The listing builds one solid part. Answer for the finished solid, in the listing's coordinates (mm). A direction names the side the tool comes from. Coordinates: 2 decimals unless noted, no trailing zeros. Order: outer loops, then holes, each group sorted by start corner. A loop starts at its lowest first (then second) coordinate and runs counter-clockwise, first axis right, second up. Notation, with made-up numbers: M 16.25,-16.75 L 36.25,-16.75 A16 cw 36.25,-11.75 Z; hole C 60,-1.5 d4. An arc over 180 degrees is marked long. One line per item, written item: value. Start each with the question number.
Q1. The part is cut by section B-B on y = 0. Give the number of separate pieces and of enclosed holes in the cut face, then the cut area to 3 significant figures.
Q2. Straight lines are drawn through the part: line 1 along X through (y, z) = (-0.25, 4.25); line 2 along X through (y, z) = (0, 1.15); line 3 along Y through (x, z) = (-16.4, -3). For each, find the intervals that lie inside material, in ascending order. Write a range as [from, to].
Q3. Determine the mould class of faces 1 (the flat face through (-4.5, 0, 4)), 2 (the flat face through (15, 0, 2)), 3 (the cylindrical face through (-15.986, 3.036, -2.751)), 4 (the flat face through (1, -5, 4)) for opening direction X: pulls with the +X half, pulls with the -X half, needs draft (parallel to the pull), parting line crosses it, or undercut.
Q4. Each of these flat-tipped pins is pushed along its axis until it touches: pin 1 Ø3 at (y, z) = (-3, -2) entering from +X; pin 2 Ø2 at (x, y) = (2, 4) entering from -Z; pin 3 Ø5 at (x, y) = (10.5, 1) entering from +Z. Where does it stop, or does it pass through?
Q5. The part is cut by section A-A on x = 10.5. Give the vertices of the cut face in (y, z).
Q6. For faces 5 (the flat face through (3, 2, -2)), 6 (the flat face through (10, -5, 4)), 7 (the cylindrical face through (6.504, -0.176, -0.986)), determine the directions among +Z, -Z, +X, -X, +Y, -Y from which every point of the face is accessible in a straight line to the end or side of a thin tool.
Q7. The part is cut by section C-C on x = -7.5. Give the vertices of the cut face in (y, z), then the cut area to 3 significant figures.
```python
from build123d import *

# Parameters (mm, degrees)
SKETCH1_W           = 30
SKETCH1_H           = 13
BOSS_EXTRUDE1_DEPTH = 5
SKETCH2_W           = 9
SKETCH2_H           = 10
SKETCH2_W_2         = 6
CUT_EXTRUDE1_DEPTH  = 3
SKETCH3_R           = 2
CUT_EXTRUDE2_DEPTH  = 5
SKETCH4_W           = 11
SKETCH4_H           = 13
BOSS_EXTRUDE2_DEPTH = 2
SKETCH5_R           = 1.15
CUT_EXTRUDE3_DEPTH  = 2
SKETCH6_R           = 4
SKETCH6_R_2         = 2
BOSS_EXTRUDE3_DEPTH = 2


with BuildPart() as part:
    # Sketch1 → Boss-Extrude1 (new body)
    with BuildSketch(Plane.XY):
        Rectangle(SKETCH1_W, SKETCH1_H)
    extrude(amount=BOSS_EXTRUDE1_DEPTH)

    # Sketch2 → Cut-Extrude1 (cut)
    with BuildSketch(Plane.XY.offset(5)):
        with Locations((-9, 0)):
            Rectangle(SKETCH2_W, SKETCH2_H)
        with Locations((1.5, 0)):
            Rectangle(SKETCH2_W, SKETCH2_H)
        with Locations((10.5, 0)):
            Rectangle(SKETCH2_W_2, SKETCH2_H)
    extrude(amount=-CUT_EXTRUDE1_DEPTH, mode=Mode.SUBTRACT)

    # Sketch3 → Cut-Extrude2 (cut)
    with BuildSketch(Plane.XY.offset(2)):
        with Locations((-9, 0)):
            Circle(SKETCH3_R)
        with Locations((1.5, 0)):
            Circle(SKETCH3_R)
        with Locations((10.5, 0)):
            Circle(SKETCH3_R)
    extrude(amount=-CUT_EXTRUDE2_DEPTH, mode=Mode.SUBTRACT)

    # Sketch4 → Boss-Extrude2 (add)
    with BuildSketch(Plane.ZY.offset(15)):
        with Locations((-0.5, 0)):
            Rectangle(SKETCH4_W, SKETCH4_H)
    extrude(amount=BOSS_EXTRUDE2_DEPTH)

    # Sketch5 → Cut-Extrude3 (cut)
    with BuildSketch(Plane(origin=(-15, 0, 0), x_dir=(0, 0, -1), z_dir=(1, 0, 0))):
        with Locations((3, 4.158153832)):
            Circle(SKETCH5_R)
        with Locations((3, -2.579108073)):
            Circle(SKETCH5_R)
    extrude(amount=-CUT_EXTRUDE3_DEPTH, mode=Mode.SUBTRACT)

    # Sketch6 → Boss-Extrude3 (add)
    with BuildSketch(Plane(origin=(0, 0, 0), x_dir=(-1, 0, 0), z_dir=(0, 0, -1))):
        with Locations(Location((-10.5, 0, 0), (0, 0, 180))):
            Circle(SKETCH6_R)
        with Locations(Location((-10.5, 0, 0), (0, 0, 180))):
            Circle(SKETCH6_R_2, mode=Mode.SUBTRACT)
        with Locations(Location((-1.5, 0, 0), (0, 0, 180))):
            Circle(SKETCH6_R)
        with Locations(Location((-1.5, 0, 0), (0, 0, 180))):
            Circle(SKETCH6_R_2, mode=Mode.SUBTRACT)
        with Locations(Location((9, 0, 0), (0, 0, 180))):
            Circle(SKETCH6_R)
        with Locations(Location((9, 0, 0), (0, 0, 180))):
            Circle(SKETCH6_R_2, mode=Mode.SUBTRACT)
    extrude(amount=BOSS_EXTRUDE3_DEPTH)


solid = part.part
```
Output:
1. separate pieces: 4
1. enclosed holes: 0
1. area: 100 mm^2
2. line 1: x = [-17, -13.5], [-4.5, -3], [6, 7.5], [13.5, 15]
2. line 2: x = [-17, -11], [-7, -0.5], [3.5, 8.5], [12.5, 15]
2. line 3: y = [-6.5, -3.73], [-1.43, 3.01], [5.31, 6.5]
3. face 1: undercut
3. face 2: pulls with the +X half
3. face 3: needs draft
3. face 4: undercut
4. pin 1: stops at x = 14.21
4. pin 2: stops at z = -2
4. pin 3: stops at z = 2
5. outline: M -6.5,0 L -4,0 L -4,-2 L -2,-2 L -2,2 L -5,2 L -5,5 L -6.5,5 Z; M 2,-2 L 4,-2 L 4,0 L 6.5,0 L 6.5,5 L 5,5 L 5,2 L 2,2 Z
6. face 5: -Z, +X, +Y, -Y
6. face 6: +Z
6. face 7: -Z
7. outline: M -6.5,0 L -3.71,0 L -3.71,-2 L -1.32,-2 L -1.32,2 L -5,2 L -5,5 L -6.5,5 Z; M 1.32,-2 L 3.71,-2 L 3.71,0 L 6.5,0 L 6.5,5 L 5,5 L 5,2 L 1.32,2 Z
7. area: 39.2 mm^2
